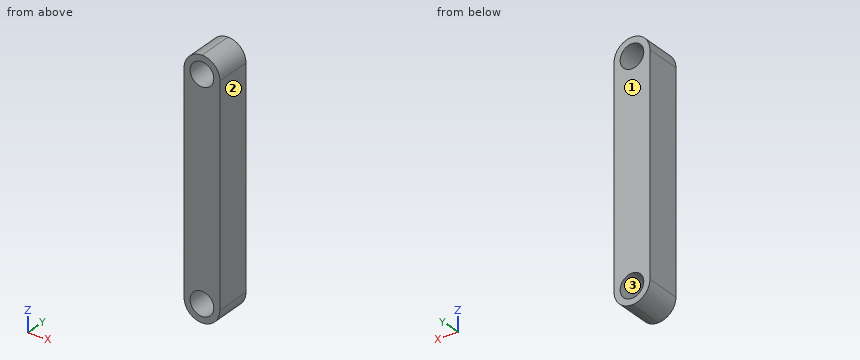
from build123d import *

# Parameters (mm, degrees)
SKETCH_2_W      = 50
SKETCH_2_H      = 350
SKETCH_2_R      = 16.5
EXTRUDE_2_DEPTH = 50
FILLET_1_R      = 25
FILLET_2_R      = 25


with BuildPart() as part:
    # 草图2 → 凸台-拉伸2 (new body)
    with BuildSketch(Plane(origin=(0, 0, 0), x_dir=(1, 0, 0), z_dir=(0, 1, 0))):
        with Locations((25, 175)):
            Rectangle(SKETCH_2_W, SKETCH_2_H)
        with Locations(Location((25, 25, 0), (0, 0, 270))):
            Circle(SKETCH_2_R, mode=Mode.SUBTRACT)
        with Locations(Location((25, 325, 0), (0, 0, 270))):
            Circle(SKETCH_2_R, mode=Mode.SUBTRACT)
    extrude(amount=EXTRUDE_2_DEPTH)

    # 圆角1
    fillet_1_edges = [part.edges().sort_by_distance(p)[0] for p in [
        (50, 25, 0),
        (0, 25, 0),
    ]]
    fillet(fillet_1_edges, radius=FILLET_1_R - 0.0001)  # a hair under: the kernel refuses the full size

    # 圆角2
    fillet_2_edges = [part.edges().sort_by_distance(p)[0] for p in [
        (50, 25, -350),
        (0, 25, -350),
    ]]
    fillet(fillet_2_edges, radius=FILLET_2_R - 0.0001)  # a hair under: the kernel refuses the full size


solid = part.part
For this review, take the finished solid that the model builds, in its own axes (mm). Face numbers are marked on the shaded views. Round coordinates to 2 decimals unless told otherwise and drop trailing zeros. Loops run counter-clockwise (first coordinate to the right, second up) from the corner with the lowest first, then second, coordinate; pieces in that order, holes last. Notation, with made-up numbers: (-10, 28) - (8, 28) arc R27 ccw to (8, 56) - close; hole circle Ø1 at (-26, 25). An arc over 180 degrees is marked (long way). One line per item, written item: value. Start each with the question number.
Item 1: For L1, parallel to X at y = 21.5, z = -25.5; L2, parallel to Z at x = 30, y = 12.5; L3, parallel to Z at x = 40, y = 38.5, list the stretches that pass through material, from the lowest coordinate up.
Item 2: The part is to be moulded in two halves that separate along X. For the marked faces 1, 2 and 3, say which applies: +X half, -X half, draft (parallel to the pull), parting line (faces both ways), or undercut.
Item 3: Take a section at B-B (x = 12.5). Give the boundary of the cut face in (y, z), plus the area to 3 significant figures.
Item 4: Take a section at C-C (x = 37). Give the boundary of the cut face in (y, z).
Item 5: Clearance check with flat-ended pins moving along their axes: pin 1 Ø4 at (x, y) = (44, 20.5) entering from +Z; pin 2 Ø2 at (x, y) = (23.5, 29.5) entering from +Z (3 decimals); pin 3 Ø3 at (x, y) = (41.5, 25) entering from +Z. State where each tip first meets the part, or that it passes through.
Item 6: Take a section at A-A (y = 17). State how many separate pieces and enclosed holes the cut face has, plus the area to 3 significant figures.
Answer below:
1. L1: x = 0 to 8.51, 41.49 to 50
1. L2: z = -349.49 to -340.72, -309.28 to -40.72, -9.28 to -0.51
1. L3: z = -345 to -331.87, -318.13 to -31.87, -18.13 to -5
2. face 1: draft
2. face 2: +X half
2. face 3: undercut
3. outline: (0, -346.65) - (50, -346.65) - (50, -335.77) - (0, -335.77) - close; (0, -314.23) - (50, -314.23) - (50, -35.77) - (0, -35.77) - close; (0, -14.23) - (50, -14.23) - (50, -3.35) - (0, -3.35) - close
3. area: 15,000 mm2
4. outline: (0, -346.93) - (50, -346.93) - (50, -336.32) - (0, -336.32) - close; (0, -313.68) - (50, -313.68) - (50, -36.32) - (0, -36.32) - close; (0, -13.68) - (50, -13.68) - (50, -3.07) - (0, -3.07) - close
5. pin 1: stops at z = -6.67
5. pin 2: stops at z = -0.005
5. pin 3: stops at z = -5
6. separate pieces: 1
6. enclosed holes: 2
6. area: 15,300 mm2
